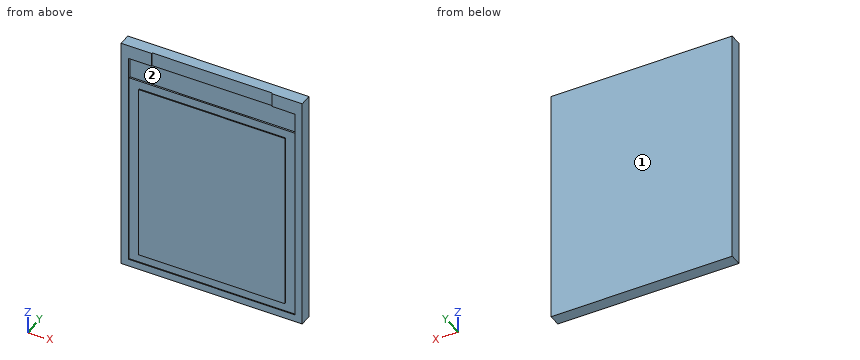
```python
from build123d import *

# Parameters (mm, degrees)
SKETCH_1_W          = 34.7
SKETCH_1_H          = 46.7
EXTRUDE_1_DEPTH     = 2.3
SKETCH_2_W          = 31.83
SKETCH_2_H          = 38.38
SKETCH_2_W_2        = 28.03
SKETCH_2_H_2        = 35.04
CUT_EXTRUDE_1_DEPTH = 0.2
SKETCH_3_W          = 31.83
SKETCH_3_H          = 4.217139833
CUT_EXTRUDE_2_DEPTH = 0.5
SKETCH_4_W          = 23.03
SKETCH_4_H          = 2.692860167
CUT_EXTRUDE_3_DEPTH = 0.2


with BuildPart() as part:
    # Эскиз1 → Бобышка-Вытянуть1 (new body)
    with BuildSketch(Plane(origin=(0, 0, 0), x_dir=(1, 0, 0), z_dir=(0, 1, 0))):
        Rectangle(SKETCH_1_W, SKETCH_1_H)
    extrude(amount=EXTRUDE_1_DEPTH)

    # Эскиз2 → Вырез-Вытянуть1 (cut)
    with BuildSketch(Plane.XZ):
        with Locations((0, -2.75)):
            Rectangle(SKETCH_2_W, SKETCH_2_H)
        with Locations((0, -2.75)):
            Rectangle(SKETCH_2_W_2, SKETCH_2_H_2, mode=Mode.SUBTRACT)
    extrude(amount=-CUT_EXTRUDE_1_DEPTH, mode=Mode.SUBTRACT)

    # Эскиз3 → Вырез-Вытянуть2 (cut)
    with BuildSketch(Plane.XZ):
        with Locations((0, 18.548569916)):
            Rectangle(SKETCH_3_W, SKETCH_3_H)
    extrude(amount=-CUT_EXTRUDE_2_DEPTH, mode=Mode.SUBTRACT)

    # Эскиз4 → Вырез-Вытянуть3 (cut)
    with BuildSketch(Plane.XZ):
        with Locations((0, 22.003569917)):
            Rectangle(SKETCH_4_W, SKETCH_4_H)
    extrude(amount=-CUT_EXTRUDE_3_DEPTH, mode=Mode.SUBTRACT)


solid = part.part
```
The listing builds one solid part. Answer for the finished solid, in the listing's coordinates (mm). Face numbers are marked on the shaded views. Coordinates: 2 decimals unless noted, no trailing zeros. Write each loop counter-clockwise with the first axis right and the second up, starting at its lowest first coordinate (ties: lowest second). Pieces come first, ordered by that corner, then holes. Notation, with made-up numbers: (22.25, 84) - (26.25, 84) arc R24 ccw to (26.25, 113) - close; hole circle Ø11 at (82, 12). An arc over 180 degrees is marked (long way). Return JSON: item names as keys, results as strings. Group by question number.
Q1. Flat-ended cylindrical pins translate along their axes: pin 1 Ø3 at (x, z) = (2, 22) entering from -Y; pin 2 Ø2 at (x, z) = (-6, 18) entering from -Y. Find the tip coordinate at first contact, or state that the pin passes through.
Q2. Find the intervals of material crossed by line 1 along X through (y, z) = (0.15, -12.5) (3 decimals); line 2 along Z through (x, y) = (12, 0.1); line 3 along Y through (x, z) = (5.5, -21), in increasing order. Write a range as [from, to].
Q3. The part is cut by section B-B on z = 20. Write down the section's boundary in (x, y) (3 decimals).
Q4. The part is cut by section C-C on x = -8. Write down the section's boundary in (y, z), and give its area (3 significant figures).
Q5. For a pull along X with two mould halves and no side action, classify the marked faces 1 and 2 as +X half, -X half, draft (parallel to the pull), parting line (faces both ways), or undercut.
Q6. The part is cut by section A-A on x = 13. Write down the section's boundary in (y, z).
Evaluation:
{
 "1": {"pin 1": "stops at y = 0.2", "pin 2": "stops at y = 0.5"},
 "2": {"line 1": "x = [-17.35, -15.915], [-14.015, 14.015], [15.915, 17.35]", "line 2": "z = [-23.35, -21.94], [-20.27, 14.77], [20.66, 23.35]", "line 3": "y = [0.2, 2.3]"},
 "3": {"outline": "(-17.35, 0) - (-15.915, 0) - (-15.915, 0.5) - (15.915, 0.5) - (15.915, 0) - (17.35, 0) - (17.35, 2.3) - (-17.35, 2.3) - close"},
 "4": {"outline": "(0, -23.35) - (2.3, -23.35) - (2.3, 23.35) - (0.2, 23.35) - (0.2, 20.66) - (0.5, 20.66) - (0.5, 16.44) - (0.2, 16.44) - (0.2, 14.77) - (0, 14.77) - (0, -20.27) - (0.2, -20.27) - (0.2, -21.94) - (0, -21.94) - close", "area": "104 mm2"},
 "5": {"face 1": "draft", "face 2": "undercut"},
 "6": {"outline": "(0, -23.35) - (2.3, -23.35) - (2.3, 23.35) - (0, 23.35) - (0, 20.66) - (0.5, 20.66) - (0.5, 16.44) - (0.2, 16.44) - (0.2, 14.77) - (0, 14.77) - (0, -20.27) - (0.2, -20.27) - (0.2, -21.94) - (0, -21.94) - close"}
}
